Read the model definition and answer for the solid it produces. Units are mm, in the model's axes. Face numbers are marked on the shaded views. A direction names the side the tool comes from. Coordinates: 2 decimals unless noted, no trailing zeros. Write each loop counter-clockwise with the first axis right and the second up, starting at its lowest first coordinate (ties: lowest second). Pieces come first, ordered by that corner, then holes. Notation, with made-up numbers: (-39, 12.25) -> (6, 12.25) arc R25 ccw to (6, 33.25) -> close; hole circle Ø1 at (59.5, -13.5). An arc over 180 degrees is marked (long way). Answer in a Markdown table with one row per item. Add a question column.
Item 1: Straight lines are drawn through the part: line 1 (Y direction, x = -5.5, z = 1.1); line 2 (Y direction, x = -10.25, z = 19); line 3 (Z direction, x = -7.5, y = -8.5). For each, find the intervals that lie inside material, in ascending order. Write a range as from..to.
Item 2: Section C-C on x = -5.5 is taken. Write down the section's boundary in (y, z).
Item 3: Which of the six approach directions +Z, -Z, +X, -X, +Y, -Y give full straight-line access (tool end or side, diameter ignored) to the marked faces 1 and 2?
Item 4: Given pin 1 Ø4 at (x, z) = (0, 21) entering from -Y; pin 2 Ø5 at (x, y) = (-5.5, 2.5) entering from +Z; pin 3 Ø1.8 at (x, y) = (5.5, -5.5) entering from -Z, each flat-ended and moving along its own axis, determine where each tip first touches the part or whether it passes through.
Item 5: Section B-B on y = -5.5 is taken. Write down the section's boundary in (x, z), then the cut area to 3 significant figures.
Item 6: Section D-D on x = 9.25 is taken. Write down the section's boundary in (y, z), then the cut area to 3 significant figures.
Item 7: Section A-A on z = 21 is taken. Write down the section's boundary in (x, y).
```python
from build123d import *

# Parameters (mm, degrees)
F0_W     = 25
F0_H     = 25
F1_DEPTH = 3
F3_D     = 3
F3_DEPTH = 15
F4_W     = 25
F4_H     = 3
F5_DEPTH = 22
F7_D     = 3


with BuildPart() as f1:
    # F0 (on Top) → F1 (new body)
    with BuildSketch(Plane.XY):
        Rectangle(F0_W, F0_H)
    extrude(amount=F1_DEPTH)

    # F3
    with Locations(Plane.XY.offset(3)):
        with Locations((5.5, 2.5), (5.5, -5.5), (-5.5, -5.5), (-5.5, 2.5)):
            Hole(F3_D / 2, depth=F3_DEPTH)

    # F4 (on face) → F5 (join)
    with BuildSketch(Plane.XY.offset(3)):
        with Locations((0, 11)):
            Rectangle(F4_W, F4_H)
    extrude(amount=F5_DEPTH)

    # F7 (through all)
    with Locations(Plane.XZ.offset(-9.5)):
        with Locations((0, 21), (0, 6)):
            Hole(F7_D / 2)


solid = f1.part
```
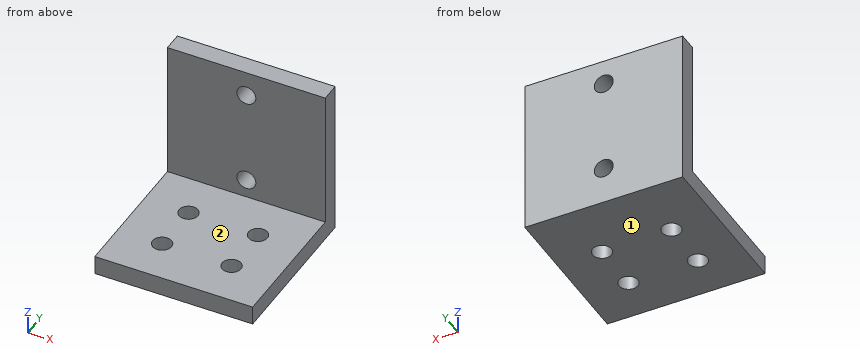
Results below:
| question | item | result |
|---|---|---|
| 1 | line 1 | y = -12.5..-7, -4..1, 4..12.5 |
| 1 | line 2 | y = 9.5..12.5 |
| 1 | line 3 | z = 0..3 |
| 2 | outline | (-12.5, 0) -> (-7, 0) -> (-7, 3) -> (-12.5, 3) -> close; (-4, 0) -> (1, 0) -> (1, 3) -> (-4, 3) -> close; (4, 0) -> (12.5, 0) -> (12.5, 25) -> (9.5, 25) -> (9.5, 3) -> (4, 3) -> close |
| 3 | face 1 | -Z, +X, -X, +Y, -Y |
| 3 | face 2 | +Z, +X, -X, -Y |
| 4 | pin 1 | stops at y = 9.5 |
| 4 | pin 2 | stops at z = 3 |
| 4 | pin 3 | passes through |
| 5 | outline | (-12.5, 0) -> (-7, 0) -> (-7, 3) -> (-12.5, 3) -> close; (-4, 0) -> (4, 0) -> (4, 3) -> (-4, 3) -> close; (7, 0) -> (12.5, 0) -> (12.5, 3) -> (7, 3) -> close |
| 5 | area | 57.0 mm2 |
| 6 | outline | (-12.5, 0) -> (12.5, 0) -> (12.5, 25) -> (9.5, 25) -> (9.5, 3) -> (-12.5, 3) -> close |
| 6 | area | 141 mm2 |
| 7 | outline | (-12.5, 9.5) -> (-1.5, 9.5) -> (-1.5, 12.5) -> (-12.5, 12.5) -> close; (1.5, 9.5) -> (12.5, 9.5) -> (12.5, 12.5) -> (1.5, 12.5) -> close |
